from build123d import *

# Parameters (mm, degrees)
SKETCH1_W           = 25.7
SKETCH1_H           = 28.5
BOSS_EXTRUDE1_DEPTH = 3
SKETCH3_W           = 5
SKETCH3_H           = 3
SKETCH3_W_2         = 2
SKETCH3_W_3         = 3
SKETCH3_H_2         = 4
CUT_EXTRUDE2_DEPTH  = 10
SKETCH2_W           = 5
SKETCH2_H           = 4.84993503
CUT_EXTRUDE3_DEPTH  = 3


with BuildPart() as part:
    # Sketch1 → Boss-Extrude1 (new body)
    with BuildSketch(Plane(origin=(0, 0, 0), x_dir=(1, 0, 0), z_dir=(0, 1, 0))):
        Rectangle(SKETCH1_W, SKETCH1_H)
    extrude(amount=BOSS_EXTRUDE1_DEPTH)

    # Sketch3 → Cut-Extrude2 (cut)
    with BuildSketch(Plane.XZ):
        with Locations((7.35, -12.75)):
            Rectangle(SKETCH3_W, SKETCH3_H)
        with Locations((-2.65, -12.75)):
            Rectangle(SKETCH3_W, SKETCH3_H)
        with Locations((-2.65, 12.75)):
            Rectangle(SKETCH3_W, SKETCH3_H)
        with Locations((7.35, 12.75)):
            Rectangle(SKETCH3_W, SKETCH3_H)
        with Locations((-10.536209453, 12.75)):
            Rectangle(SKETCH3_W_2, SKETCH3_H)
        with Locations((-10.536209453, -12.75)):
            Rectangle(SKETCH3_W_2, SKETCH3_H)
        with Locations((11.35, -4.5)):
            Rectangle(SKETCH3_W_3, SKETCH3_H_2)
        with Locations((11.35, 4.5)):
            Rectangle(SKETCH3_W_3, SKETCH3_H_2)
    extrude(amount=-CUT_EXTRUDE2_DEPTH, mode=Mode.SUBTRACT)

    # Sketch2 → Cut-Extrude3 (cut)
    with BuildSketch(Plane.XZ):
        with Locations((-7.35, -13.674967515)):
            Rectangle(SKETCH2_W, SKETCH2_H)
        with Locations((-7.35, 13.674967515)):
            Rectangle(SKETCH2_W, SKETCH2_H)
    extrude(amount=-CUT_EXTRUDE3_DEPTH, mode=Mode.SUBTRACT)


solid = part.part
Here's how the part is built. I have some questions about the finished solid (model axes, mm). A direction names the side the tool comes from. Round coordinates to 2 decimals unless told otherwise and drop trailing zeros. Order: outer loops, then holes, each group sorted by start corner. A loop starts at its lowest first (then second) coordinate and runs counter-clockwise, first axis right, second up. Notation, with made-up numbers: M -19,13.25 L -9,13.25 A15 ccw -9,29.25 Z; hole C 76.25,20 d11. An arc over 180 degrees is marked long. Return JSON: item names as keys, results as strings. Group by question number.
1. If we mould it in two halves opening along X, with no side actions, what happens to faces 1 (the face through (7, 1, 11.25)), 2 (the face through (12.85, 1, -10)), 3 (the face through (2, 1, 14.25))? For each: pulls with the +X half, pulls with the -X half, needs draft (parallel to the pull), parting line crosses it, or undercut.
2. If we section it at B-B on y = 1: List the corners of the cut face in (x, z) for me.
3. If we section it at D-D on z = -4.75: List the corners of the cut face in (x, y) for me.
4. Please list where these lines run through material, in increasing order: probe 1 along X at (y, z) = (1.6, 13); probe 2 along Z at (x, y) = (-11, 0.65); probe 3 along X at (y, z) = (0.75, -4.5).
5. If we section it at C-C on x = 7.5: List the corners of the cut face in (y, z) for me.
6. I'm going to push flat-ended pins straight in: pin 1 Ø0.9 at (x, y) = (7, 1.5) entering from -Z; pin 2 Ø4 at (x, z) = (8.5, -2) entering from -Y. Where does each tip first touch, or does it pass through?
7. On a 3-axis mill with a long thin cutter (end or side, diameter ignored), from which of +Z, -Z, +X, -X, +Y, -Y can I reach the whole of each face in a straight line? I mean faces 4 (the face through (11, 1, 2.5)), 5 (the face through (-11.536, 1, -13)), 6 (the face through (4.85, 1, 13)). Say none if no direction works.
8. If we section it at A-A on z = 12.75: List the corners of the cut face in (x, y) for me, then the cut area to 3 significant figures.
Reply:
{
 "1": {"face 1": "undercut", "face 2": "pulls with the +X half", "face 3": "needs draft"},
 "2": {"outline": "M -12.85,-14.25 L -11.54,-14.25 L -11.54,-11.25 L -0.15,-11.25 L -0.15,-14.25 L 4.85,-14.25 L 4.85,-11.25 L 9.85,-11.25 L 9.85,-14.25 L 12.85,-14.25 L 12.85,-6.5 L 9.85,-6.5 L 9.85,-2.5 L 12.85,-2.5 L 12.85,2.5 L 9.85,2.5 L 9.85,6.5 L 12.85,6.5 L 12.85,14.25 L 9.85,14.25 L 9.85,11.25 L 4.85,11.25 L 4.85,14.25 L -0.15,14.25 L -0.15,11.25 L -11.54,11.25 L -11.54,14.25 L -12.85,14.25 Z"},
 "3": {"outline": "M -12.85,0 L 9.85,0 L 9.85,3 L -12.85,3 Z"},
 "4": {"probe 1": "-12.85 to -11.54, -0.15 to 4.85, 9.85 to 12.85", "probe 2": "-11.25 to 11.25", "probe 3": "-12.85 to 9.85"},
 "5": {"outline": "M 0,-11.25 L 3,-11.25 L 3,11.25 L 0,11.25 Z"},
 "6": {"pin 1": "z = -11.25", "pin 2": "y = 0"},
 "7": {"face 4": "+X, +Y, -Y", "face 5": "-Z, +Y, -Y", "face 6": "+Z, +Y, -Y"},
 "8": {"outline": "M -12.85,0 L -11.54,0 L -11.54,3 L -12.85,3 Z; M -0.15,0 L 4.85,0 L 4.85,3 L -0.15,3 Z; M 9.85,0 L 12.85,0 L 12.85,3 L 9.85,3 Z", "area": "27.9 mm^2"}
}
